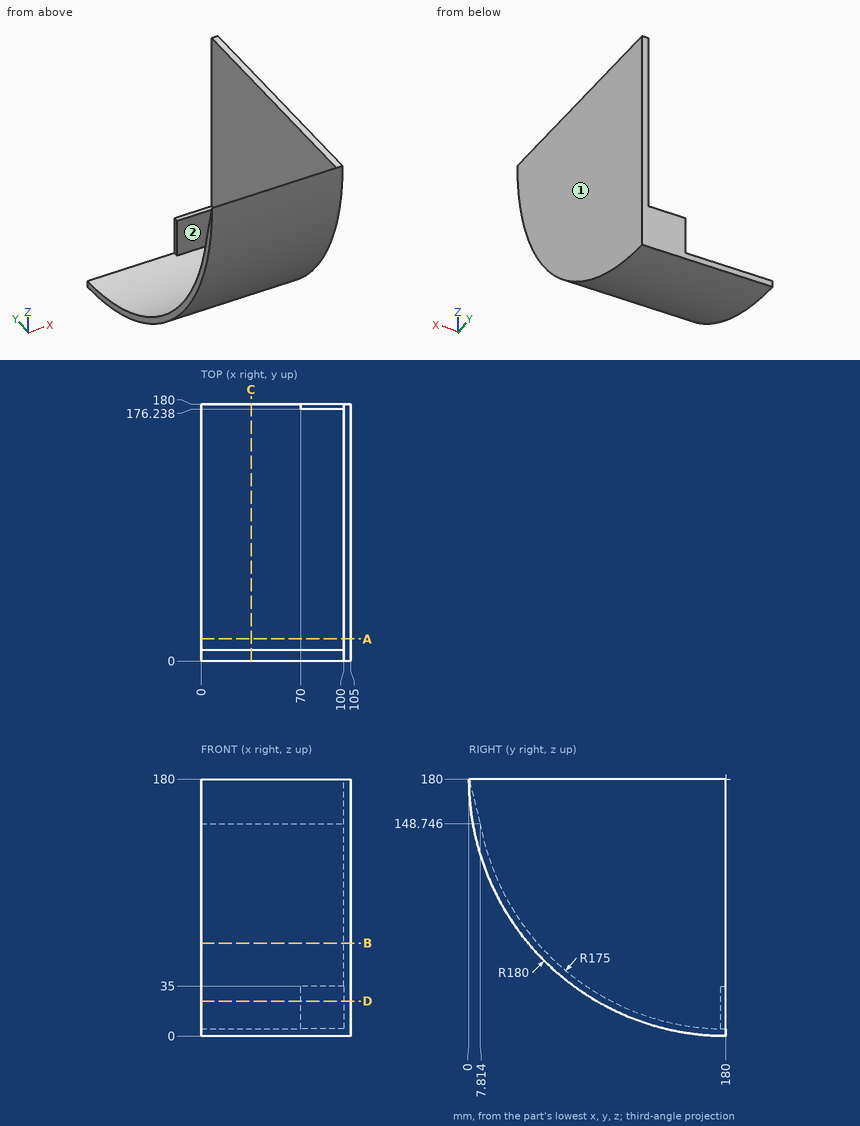
Here's the drawing with two shaded views (mm, measured from the low corner). I have some questions. A direction names the side the tool comes from. Give positions to 0.01 mm unless a question says otherwise; leave off trailing zeros. Loops run counter-clockwise (first coordinate to the right, second up) from the corner with the lowest first, then second, coordinate; pieces in that order, holes last. Notation, with made-up numbers: (53, -11.75) - (66, -11.75) arc R26 cw to (66, 8.25) - close; hole circle Ø1 at (-7.75, -27.5). An arc over 180 degrees is marked (long way). Answer in a Markdown table with one row per item. Add a question column.
Q1. For pin 1 (1 mm diameter, centred on x = 63, y = 147.5, fed in from +Z); pin 2 (6 mm diameter, centred on x = 49.5, y = 29, fed in from +Z); pin 3 (1 mm diameter, centred on x = 45, z = 33, fed in from +Y) (1 decimal), each with a flat end and sliding along its axis, tell me the tip position at first contact or that it passes through.
Q2. If we section it at A-A (y = 15.5): List the corners of the cut face in (x, z) for me (1 decimal), plus the area to 3 significant figures.
Q3. Which directions (+Z, -Z, +X, -X, +Y, -Y) give clear straight access to the entire face, cutting with the end or side of a thin tool? Please do the marked faces 1 and 2.
Q4. If we section it at D-D (z = 24.5): List the corners of the cut face in (x, y) for me, plus the area to 3 significant figures.
Q5. If we section it at B-B (z = 65): List the corners of the cut face in (x, y) for me.
Q6. If we section it at C-C (x = 35): List the corners of the cut face in (y, z) for me (1 decimal).
Q7. Please list where these lines run through material, in increasing order: L1, parallel to X at y = 107, z = 28; L2, parallel to Z at x = 12.5, y = 54.5 (1 decimal); L3, parallel to Z at x = 72.5, y = 100 (1 decimal). Write a range as from..to.
The answers:
| question | item | result |
|---|---|---|
| 1 | pin 1 | stops at z = 8.14 |
| 1 | pin 2 | stops at z = 96.88 |
| 1 | pin 3 | stops at y = 85.8 |
| 2 | outline | (0, 106.9) - (105, 106.9) - (105, 180) - (100, 180) - (100, 120.3) - (0, 120.3) - close |
| 2 | area | 1,700 mm^2 |
| 3 | face 1 | +Z, -Z, +X, +Y, -Y |
| 3 | face 2 | +Z, -X |
| 4 | outline | (0, 89.34) - (105, 89.34) - (105, 180) - (70, 180) - (70, 176.24) - (100, 176.24) - (100, 99.72) - (0, 99.72) - close |
| 4 | area | 1,600 mm^2 |
| 5 | outline | (0, 41.53) - (105, 41.53) - (105, 180) - (100, 180) - (100, 48.09) - (0, 48.09) - close |
| 6 | outline | (0, 180) arc R180 ccw to (180, 0) - (180, 5) arc R175 cw to (7.8, 148.7) - close |
| 7 | L1 | x = 100..105 |
| 7 | L2 | z = 51..58 |
| 7 | L3 | z = 18.8..24.4 |
